from build123d import *

# Parameters (mm, degrees)
BOSS_EXTRUDE1_START                               = -12.7
BOSS_EXTRUDE1_DEPTH                               = 12.7
CUT_EXTRUDE1_DEPTH                                = 6799.247512927
BOSS_EXTRUDE2_DEPTH                               = 6.35
BOSS_EXTRUDE3_DEPTH                               = 19.05
CUT_EXTRUDE2_REACH                                = 3294.662
SKETCH5_W                                         = 19.05
SKETCH5_H                                         = 70.738300655
F_8_START                                         = 79
F_8_CLEARANCE_HOLE1_OUTLINE_R                     = 2.45745
F_8_CLEARANCE_HOLE1_DEPTH                         = 21
SKETCH22_W                                        = 19.05
SKETCH22_H                                        = 109.611311192
CUT_EXTRUDE3_DEPTH                                = 20.02562
CSK_FOR_8_FLAT_HEAD_MACHINE_SCREW_100_D           = 4.9149
CSK_FOR_8_FLAT_HEAD_MACHINE_SCREW_100_CSINK_D     = 8.4328
CSK_FOR_8_FLAT_HEAD_MACHINE_SCREW_100_CSINK_ANGLE = 100
CUT_EXTRUDE4_DEPTH                                = 6764.722428504
FILLET1_R                                         = 203.2
HOLE6_D                                           = 3.175
HOLE6_DEPTH                                       = 31.75
HOLE6_CSINK_D                                     = 10.16
HOLE6_CSINK_ANGLE                                 = 82
HOLE6_TIP                                         = 0.953866233
CSK_FOR_6_FLAT_HEAD_MACHINE_SCREW1_D              = 3.7973
CSK_FOR_6_FLAT_HEAD_MACHINE_SCREW1_CSINK_D        = 7.0866
CSK_FOR_6_FLAT_HEAD_MACHINE_SCREW1_CSINK_ANGLE    = 82
CSK_FOR_4_FLAT_HEAD_MACHINE_SCREW1_D              = 3.2639
CSK_FOR_4_FLAT_HEAD_MACHINE_SCREW1_CSINK_D        = 5.715
CSK_FOR_4_FLAT_HEAD_MACHINE_SCREW1_CSINK_ANGLE    = 82
CSK_FOR_2_FLAT_HEAD_MACHINE_SCREW1_D              = 2.4384
CSK_FOR_2_FLAT_HEAD_MACHINE_SCREW1_CSINK_D        = 4.3688
CSK_FOR_2_FLAT_HEAD_MACHINE_SCREW1_CSINK_ANGLE    = 82
CUT_EXTRUDE6_DEPTH                                = 15.875


with BuildPart() as part:
    # Boss-Extrude1: read off the stored shape, not the designer's step
    # Boss-Extrude1 outline → Boss-Extrude1 (new body)
    with BuildSketch(Plane(origin=(99.06, 0, 0), x_dir=(0, 0, -1), z_dir=(1, 0, 0)).offset(BOSS_EXTRUDE1_START)):
        Polygon((-3048.635, 5823.580065533), (-3048.635, 5817.939621245), (-3279.272122652, 5764.692845932), (-3270.701487481, 5727.569346464), (-2759.71, 5845.541026859), (-2759.71, 5955.030000144), (-2807.335, 5955.030000144), (-2804.426960815, 5949.385019356), align=None)
    extrude(amount=BOSS_EXTRUDE1_DEPTH)

    # Sketch2 → Cut-Extrude1 (cut, through all)
    with BuildSketch(Plane(origin=(99.06, 0, 0), x_dir=(0, 0, -1), z_dir=(1, 0, 0))):
        Polygon((-3279.272122652, 5764.692845932), (-3048.635, 5817.939621245), (-3048.635, 5814.764621245), (-3278.576208456, 5761.678510384), align=None)
    extrude(amount=-CUT_EXTRUDE1_DEPTH, mode=Mode.SUBTRACT)

    # Sketch3 → Boss-Extrude2 (add)
    with BuildSketch(Plane.ZY.offset(-86.36)):
        Polygon((3278.576208456, 5761.678510384), (3048.635, 5814.764621245), (3048.635, 5823.580065533), (2804.426960815, 5949.385019356), (2807.335, 5955.030000144), (2759.71, 5955.030000144), (2759.71, 5845.541026859), (3270.701487481, 5727.569346464), align=None)
    extrude(amount=BOSS_EXTRUDE2_DEPTH)

    # Sketch4 → Boss-Extrude3 (add, through all)
    with BuildSketch(Plane.ZY.offset(-80.01)):
        Polygon((2759.71, 5845.541026859), (3270.701487481, 5727.569346464), (3252.406488556, 5648.325), (2759.71, 5648.325), align=None)
    extrude(amount=-BOSS_EXTRUDE3_DEPTH)

    # Sketch5 → Cut-Extrude2 (cut, up to next)
    with BuildSketch(Plane(origin=(0, 5935.980000144, 0), x_dir=(1, 0, 0), z_dir=(0, 1, 0)), mode=Mode.PRIVATE) as cut_extrude2_sk1:
        with Locations((89.535, -2795.079150328)):
            Rectangle(SKETCH5_W, SKETCH5_H)
    cut_extrude2_tool1 = extrude(cut_extrude2_sk1.sketch, amount=CUT_EXTRUDE2_REACH, mode=Mode.PRIVATE) & part.part
    add(cut_extrude2_tool1.solids().sort_by_distance((89.535, 5935.98, 2795.07915))[0], mode=Mode.SUBTRACT)

    # #8 Clearance Hole1: read off the stored shape, not the designer's step
    # #8 Clearance Hole1 outline → #8 Clearance Hole1 (cut)
    with BuildSketch(Plane.YZ.offset(F_8_START)):
        with Locations((5737.333926367, 3143.899589677)):
            Circle(F_8_CLEARANCE_HOLE1_OUTLINE_R)
        with Locations((5756.611506802, 3133.589577954)):
            Circle(F_8_CLEARANCE_HOLE1_OUTLINE_R)
        with Locations((5729.634798773, 3255.030012286)):
            Circle(F_8_CLEARANCE_HOLE1_OUTLINE_R)
    extrude(amount=F_8_CLEARANCE_HOLE1_DEPTH, mode=Mode.SUBTRACT)

    # 8 Clearance Hole1 2 outline → 8 Clearance Hole1 2 (revolve, cut)
    with BuildSketch(Plane(origin=(89.535, 6106.319771445, 1409.755000067), x_dir=(1, 0, 0), z_dir=(0, 0.9743700647852487, 0.2249510543438069))):
        Polygon((0.99187, -1879.400856936), (0, -1878.804881314), (0, -1898.450856936), (0.99187, -1898.450856936), align=None)
    revolve(axis=Axis((89.535, 6106.319771445, 1409.755000067), (0, 0.2249510543438069, -0.9743700647852487)), mode=Mode.SUBTRACT)

    # 8 Clearance Hole1 3 outline → 8 Clearance Hole1 3 (revolve, cut)
    with BuildSketch(Plane(origin=(89.535, 6163.988032626, 1423.068767212), x_dir=(1, 0, 0), z_dir=(0, 0.9743700647852487, 0.2249510543438069))):
        Polygon((0.99187, -1879.400856936), (0, -1878.804881314), (0, -1898.450856936), (0.99187, -1898.450856936), align=None)
    revolve(axis=Axis((89.535, 6163.988032626, 1423.068767212), (0, 0.2249510543438069, -0.9743700647852487)), mode=Mode.SUBTRACT)

    # Sketch22 → Cut-Extrude3 (cut)
    with BuildSketch(Plane(origin=(0, 5935.980000144, 0), x_dir=(1, 0, 0), z_dir=(0, 1, 0))):
        with Locations((89.535, -2814.515655596)):
            Rectangle(SKETCH22_W, SKETCH22_H)
    extrude(amount=-CUT_EXTRUDE3_DEPTH, mode=Mode.SUBTRACT)

    # CSK for #8 Flat Head Machine Screw (100)1 (through all)
    with Locations(Plane(origin=(99.06, 0, 0), x_dir=(0, 0, -1), z_dir=(1, 0, 0))):
        with Locations((-3222.137837611, 5760.045015031), (-3087.184948706, 5791.20134438), (-3038.796108056, 5817.934011474), (-2772.41, 5887.379380546)):
            CounterSinkHole(CSK_FOR_8_FLAT_HEAD_MACHINE_SCREW_100_D / 2, CSK_FOR_8_FLAT_HEAD_MACHINE_SCREW_100_CSINK_D / 2, counter_sink_angle=CSK_FOR_8_FLAT_HEAD_MACHINE_SCREW_100_CSINK_ANGLE)

    # Sketch26 → Cut-Extrude4 (cut, through all)
    with BuildSketch(Plane(origin=(99.06, 0, 0), x_dir=(0, 0, -1), z_dir=(1, 0, 0))):
        Polygon((-3252.406488556, 5648.325), (-2759.71, 5648.325), (-2759.71, 5827.054380546), (-2857.340029902, 5827.054380546), (-3110.151425601, 5681.093653185), (-3255.263366946, 5660.699499823), align=None)
    extrude(amount=-CUT_EXTRUDE4_DEPTH, mode=Mode.SUBTRACT)

    # Fillet1
    fillet1_edges = [part.edges().sort_by_distance(p)[0] for p in [
        (89.535, 5681.093653185, 3110.151425601),
        (89.535, 5827.054380546, 2857.340029902),
    ]]
    fillet(fillet1_edges, radius=FILLET1_R)

    # Hole6
    with Locations(Plane(origin=(99.06, 0, 0), x_dir=(0, 0, -1), z_dir=(1, 0, 0))):
        with Locations((-2778.76, 5836.579380546), (-2842.26, 5836.579380546)):
            CounterSinkHole(HOLE6_D / 2, HOLE6_CSINK_D / 2, depth=HOLE6_DEPTH, counter_sink_angle=HOLE6_CSINK_ANGLE)
            with Locations((0, 0, -(HOLE6_DEPTH + HOLE6_TIP / 2))):  # 118° drill point
                Cone(0, HOLE6_D / 2, HOLE6_TIP, mode=Mode.SUBTRACT)

    # CSK for #6 Flat Head Machine Screw1 (through all)
    with Locations(Plane(origin=(99.06, 0, 0), x_dir=(0, 0, -1), z_dir=(1, 0, 0))):
        with Locations((-2873.705975086, 5877.154772353)):
            CounterSinkHole(CSK_FOR_6_FLAT_HEAD_MACHINE_SCREW1_D / 2, CSK_FOR_6_FLAT_HEAD_MACHINE_SCREW1_CSINK_D / 2, counter_sink_angle=CSK_FOR_6_FLAT_HEAD_MACHINE_SCREW1_CSINK_ANGLE)

    # CSK for #4 Flat Head Machine Screw1 (through all)
    with Locations(Plane(origin=(99.06, 0, 0), x_dir=(0, 0, -1), z_dir=(1, 0, 0))):
        with Locations((-2928.787214128, 5863.882760898), (-2899.887388336, 5882.819970608)):
            CounterSinkHole(CSK_FOR_4_FLAT_HEAD_MACHINE_SCREW1_D / 2, CSK_FOR_4_FLAT_HEAD_MACHINE_SCREW1_CSINK_D / 2, counter_sink_angle=CSK_FOR_4_FLAT_HEAD_MACHINE_SCREW1_CSINK_ANGLE)

    # CSK for #2 Flat Head Machine Screw1 (through all)
    with Locations(Plane(origin=(99.06, 0, 0), x_dir=(0, 0, -1), z_dir=(1, 0, 0))):
        with Locations((-2939.003662809, 5819.981482761), (-2946.198895696, 5843.372904772)):
            CounterSinkHole(CSK_FOR_2_FLAT_HEAD_MACHINE_SCREW1_D / 2, CSK_FOR_2_FLAT_HEAD_MACHINE_SCREW1_CSINK_D / 2, counter_sink_angle=CSK_FOR_2_FLAT_HEAD_MACHINE_SCREW1_CSINK_ANGLE)

    # Sketch36 → Cut-Extrude6 (cut)
    with BuildSketch(Plane.ZY.offset(-80.01)):
        with BuildLine():
            Line((3271.237867638, 5763.372699854), (3258.863367816, 5766.229578244))
            Line((3258.863367816, 5766.229578244), (3257.43492862, 5760.042328333))
            ThreePointArc((3257.43492862, 5760.042328333), (3257.836000871, 5757.645615071), (3259.814333979, 5756.23448378))
            Line((3259.814333979, 5756.23448378), (3266.00158389, 5754.806044585))
            ThreePointArc((3266.00158389, 5754.806044585), (3268.398297151, 5755.207116835), (3269.809428443, 5757.185449943))
            Line((3269.809428443, 5757.185449943), (3271.237867638, 5763.372699854))
        make_face()
    extrude(amount=-CUT_EXTRUDE6_DEPTH, mode=Mode.SUBTRACT)


solid = part.part
Design review of the part built by this model. Coordinates are the model's own, in mm. A direction names the side the tool comes from. Give positions to 0.01 mm unless a question says otherwise; leave off trailing zeros. Write each loop counter-clockwise with the first axis right and the second up, starting at its lowest first coordinate (ties: lowest second). Pieces come first, ordered by that corner, then holes. Notation, with made-up numbers: M -1,88 L 38,88 A36 ccw 38,124 Z; hole C -15.5,-39 d4. An arc over 180 degrees is marked long. Answer as a JSON object with one key per item and string values. Group by question number.
1) We need section B-B (z = 2796.5). Give the boundary of the cut face in (x, y), and give its area (3 significant figures).
2) Tool access review of faces 5 (the face through (90, 5819, 3048.635)), 6 (the face through (89, 5915.954, 2814)), 7 (the face through (90, 5827.054, 2781)): name each direction out of +Z, -Z, +X, -X, +Y, -Y from which nothing blocks a thin tool from reaching the whole face with its end or side.
3) Mouldability with a two-part tool opening along Z and no side actions: class faces 1 (the face through (95.885, 5761, 3264)), 2 (the face through (89.4, 5684.51, 3111.91)), 3 (the face through (99.06, 5790, 3023)), 4 (the face through (89.668, 5869.121, 2960.233)) as released by +Z, released by -Z, zero draft, split by the parting line, or undercut.
4) Clearance check with flat-ended pins moving along their axes: pin 1 Ø1.5 at (x, y) = (93, 5796) entering from -Z; pin 2 Ø4 at (y, z) = (5756.61, 3133.59) entering from -X; pin 3 Ø8 at (y, z) = (5791.2, 3087.18) entering from +X; pin 4 Ø10 at (x, z) = (97, 3183) entering from -Y. State where each tip first meets the part, or that it passes through.
5) We need section A-A (y = 5897). Give the boundary of the cut face in (x, z), and give its area (3 significant figures).
6) For line 1 along Z through (x, y) = (81.75, 5757); line 2 along Y through (x, z) = (86, 3087.5); line 3 along Y through (x, z) = (81, 3088.5), list the stretches that pass through material, from the lowest coordinate up.
Answer key:
{
 "1": {"outline": "M 80.01,5827.05 L 99.06,5827.05 L 99.06,5915.95 L 80.01,5915.95 Z", "area": "1,690 mm²"},
 "2": {"face 5": "+Z, +X, -X, +Y", "face 6": "+Z, -Z, +X, -X, +Y", "face 7": "-Z, +X, -X, -Y"},
 "3": {"face 1": "undercut", "face 2": "released by -Z", "face 3": "zero draft", "face 4": "released by +Z"},
 "4": {"pin 1": "stops at z = 2909.83", "pin 2": "passes through", "pin 3": "stops at x = 98.88", "pin 4": "stops at y = 5670.15"},
 "5": {"outline": "M 80.01,2759.71 L 99.06,2759.71 L 99.06,2906.11 L 80.01,2906.11 Z", "area": "2,790 mm²"},
 "6": {"line 1": "z = 2978.68 to 3131.16, 3136.02 to 3258.37, 3269.76 to 3277.5", "line 2": "y = 5694.66 to 5788.76, 5793.64 to 5805.79", "line 3": "y = 5694.17 to 5789.13, 5793.28 to 5805.56"}
}
